```python
from build123d import *

# Parameters (mm, degrees)
F1_DEPTH = 1
F3_DEPTH = 5
F5_DEPTH = 5
F6_W     = 7
F6_H     = 4
F7_DEPTH = 1


with BuildPart() as f1:
    # F0 (on Top) → F1 (new body)
    with BuildSketch(Plane.XY):
        with BuildLine():
            Line((-33.65, -25), (40, -25))
            Line((40, -25), (40, 18.65))
            ThreePointArc((40, 18.65), (38.140128, 23.140128), (33.65, 25))
            Line((33.65, 25), (-40, 25))
            Line((-40, 25), (-40, -18.65))
            ThreePointArc((-40, -18.65), (-38.140128, -23.140128), (-33.65, -25))
        make_face()
    extrude(amount=F1_DEPTH)

    # F2 (on face) → F3 (join)
    with BuildSketch(Plane(origin=(0, 0, 0), x_dir=(1, 0, 0), z_dir=(0, 0, -1))):
        with BuildLine():
            Line((39, 24), (-33.65, 24))
            ThreePointArc((-33.65, 24), (-37.433021, 22.433021), (-39, 18.65))
            Line((-39, 18.65), (-39, -24))
            Line((-39, -24), (33.65, -24))
            ThreePointArc((33.65, -24), (37.433021, -22.433021), (39, -18.65))
            Line((39, -18.65), (39, 24))
        make_face()
    extrude(amount=F3_DEPTH)

    # F4 (on face) → F5 (cut)
    with BuildSketch(Plane(origin=(0, 0, -5), x_dir=(1, 0, 0), z_dir=(0, 0, -1))):
        with BuildLine():
            Line((-38, 18.65), (-38, -23))
            Line((-38, -23), (33.65, -23))
            ThreePointArc((33.65, -23), (36.725914, -21.725914), (38, -18.65))
            Line((38, -18.65), (38, 23))
            Line((38, 23), (-33.65, 23))
            ThreePointArc((-33.65, 23), (-36.725914, 21.725914), (-38, 18.65))
        make_face()
    extrude(amount=-F5_DEPTH, mode=Mode.SUBTRACT)

    # F6 (on face) → F7 (cut, through all)
    with BuildSketch(Plane.YZ.offset(39)):
        with Locations((-6, -3)):
            Rectangle(F6_W, F6_H)
    extrude(amount=-F7_DEPTH, mode=Mode.SUBTRACT)


solid = f1.part
```
Geometry: final body of the model. Coordinates: model frame, mm. A direction names the side the tool comes from. Coordinates: 2 decimals unless noted, no trailing zeros. Order: outer loops, then holes, each group sorted by start corner. A loop starts at its lowest first (then second) coordinate and runs counter-clockwise, first axis right, second up. Notation, with made-up numbers: (-14, 41.5) - (-10, 41.5) arc R20 cw to (-10, 50.5) - close; hole circle Ø1 at (-8.5, -0.75). An arc over 180 degrees is marked (long way). Return JSON: item names as keys, results as strings. Group by question number.
1. Cut plane A-A (z = -3.1). Output: boundary loops of the cut face in (x, y), plus the area to 3 significant figures.
2. Material intervals for line 1 along Y through (x, z) = (24, -1.5); line 2 along X through (y, z) = (9.5, -0.65); line 3 along Z through (x, y) = (-36, 18.5), sorted ascending. Write a range as [from, to].
3. Cut plane C-C (y = 16.5). Output: boundary loops of the cut face in (x, z).
4. Pull-direction query (Y, two-part tool) for faces 4 (the face through (-39, 2, -2)), 5 (the face through (37.391, 22.474, -2.465)), 6 (the face through (-1, 0, 0)), 7 (the face through (-37.391, -22.474, -2.465)); classes: pulls with the +Y half, pulls with the -Y half, needs draft (parallel to the pull), parting line crosses it, or undercut.
5. Set-up query: faces 1 (the face through (3, -24, -2)), 2 (the face through (-3, 24, -2)), 3 (the face through (39, -2, -2)). Return all of +Z, -Z, +X, -X, +Y, -Y with unobstructed straight access to the full face (end or side cutting, diameter ignored); none if empty.
6. Cut plane B-B (x = -17). Output: boundary loops of the cut face in (y, z).
7. Pin query (flat end, axial travel): pin 1 (0.8 mm diameter, centred on x = 38.5, z = -2.5, fed in from +Y); pin 2 (1.5 mm diameter, centred on y = -2, z = -3, fed in from -X); pin 3 (25 mm diameter, centred on x = 13.5, y = 8, fed in from -Z). Return the tip coordinate at first contact, or that it passes through.
Resolved:
{
 "1": {"outline": "(-39, -18.65) arc R5.35 ccw to (-33.65, -24) - (39, -24) - (39, -9.5) - (38, -9.5) - (38, -23) - (-33.65, -23) arc R4.35 cw to (-38, -18.65) - (-38, 23) - (33.65, 23) arc R4.35 cw to (38, 18.65) - (38, -2.5) - (39, -2.5) - (39, 18.65) arc R5.35 ccw to (33.65, 24) - (-39, 24) - close", "area": "237 mm²"},
 "2": {"line 1": "y = [-24, -23], [23, 24]", "line 2": "x = [-39, -38], [38, 39]", "line 3": "z = [0, 1]"},
 "3": {"outline": "(-40, 0) - (-39, 0) - (-39, -5) - (-38, -5) - (-38, 0) - (38, 0) - (38, -5) - (39, -5) - (39, 0) - (40, 0) - (40, 1) - (-40, 1) - close"},
 "4": {"face 4": "needs draft", "face 5": "pulls with the +Y half", "face 6": "undercut", "face 7": "pulls with the -Y half"},
 "5": {"face 1": "-Z, +X, -X, -Y", "face 2": "-Z, +X, -X, +Y", "face 3": "-Z, +X, +Y, -Y"},
 "6": {"outline": "(-25, 0) - (-24, 0) - (-24, -5) - (-23, -5) - (-23, 0) - (23, 0) - (23, -5) - (24, -5) - (24, 0) - (25, 0) - (25, 1) - (-25, 1) - close"},
 "7": {"pin 1": "stops at y = 21.62", "pin 2": "stops at x = -39", "pin 3": "stops at z = 0"}
}
